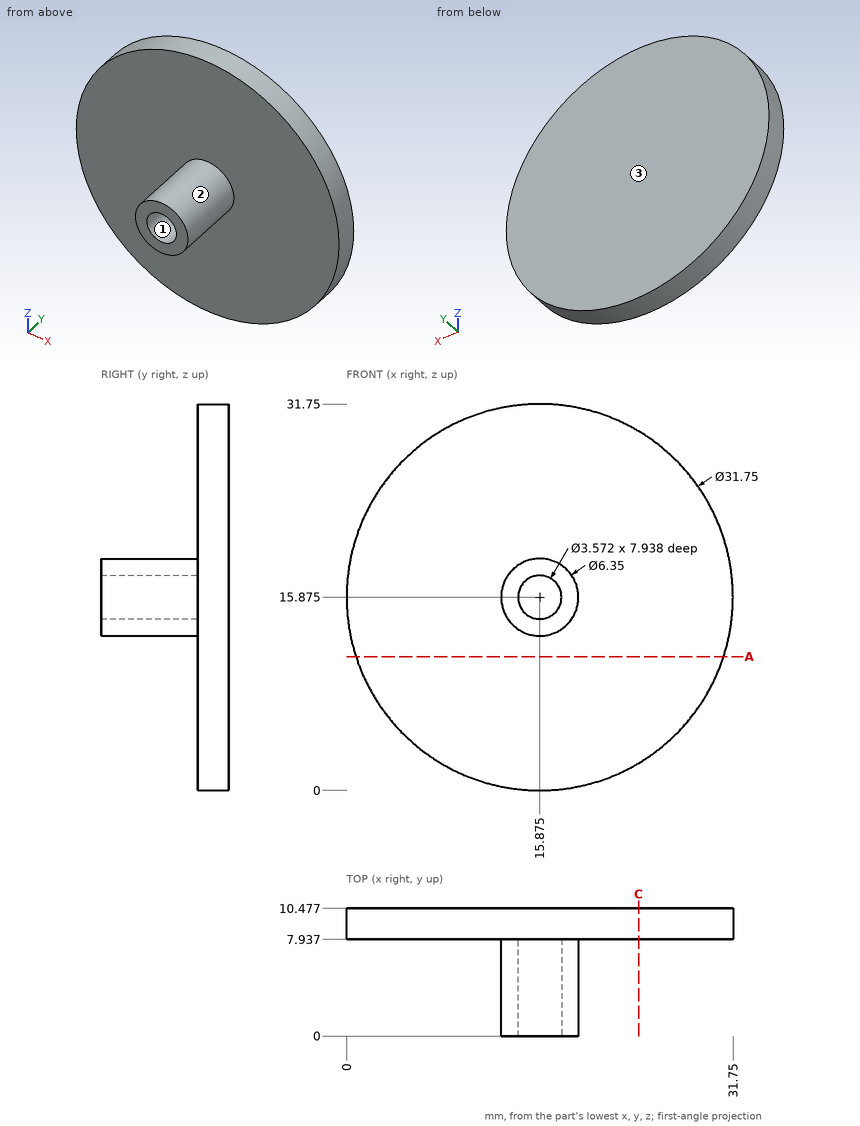
Job drawing, mm, ordinate dimensions from the low corner. One solid piece. Round coordinates to 2 decimals unless told otherwise and drop trailing zeros. Write each loop counter-clockwise with the first axis right and the second up, starting at its lowest first coordinate (ties: lowest second). Pieces come first, ordered by that corner, then holes. Notation, with made-up numbers: (40, 13.25) -> (45, 13.25) arc R22 ccw to (45, 40.25) -> close; hole circle Ø7 at (85, 84.25). An arc over 180 degrees is marked (long way). Answer as CSV lines item,"result".
1. Slice it at C-C, the plane x = 24. List the corners of the cut face in (y, z).
Resolved:
outline,"(7.94, 2.24) -> (10.48, 2.24) -> (10.48, 29.51) -> (7.94, 29.51) -> close"
2. Drill centre lines: line 1 (Z direction, x = 16, y = 3.5); line 2 (Y direction, x = 26.5, z = 23); line 3 (X direction, y = 2.25, z = 14.5) (1 decimal). Where is each one in solid material? Low to high.
Resolved:
line 1,"12.7 to 14.09, 17.66 to 19.05"
line 2,"7.94 to 10.48"
line 3,"13 to 14.7, 17 to 18.7"
3. Pin check, flat tips, straight feed: pin 1 Ø3 at (x, y) = (11, 9.5) entering from -Z; pin 2 Ø1.8 at (x, z) = (16, 16) entering from -Y; pin 3 Ø1 at (y, z) = (8.5, 3.5) entering from +X; pin 4 Ø5 at (x, y) = (5, 3) entering from +Z. Stop position of each tip, or through.
Resolved:
pin 1,"z = 0.36"
pin 2,"y = 7.94"
pin 3,"x = 26.41"
pin 4,"through"
4. Slice it at A-A, the plane z = 11. List the corners of the cut face in (x, y).
Resolved:
outline,"(0.77, 7.94) -> (30.98, 7.94) -> (30.98, 10.48) -> (0.77, 10.48) -> close"
5. Mould opens along Z. For the marked faces 1, 2 and 3 say: +Z half, -Z half, draft (parallel to the pull), parting line (faces both ways), or undercut.
Resolved:
face 1,"undercut"
face 2,"parting line"
face 3,"draft"
